from build123d import *

# Parameters (mm, degrees)
F0_W     = 150
F0_H     = 50
F1_DEPTH = 4
F3_D     = 5
F4_R     = 5
F5_SIZE  = 2


with BuildPart() as f1:
    # F0 (on Top) → F1 (new body)
    with BuildSketch(Plane.XY):
        Rectangle(F0_W, F0_H)
    extrude(amount=F1_DEPTH)

    # F3 (through all)
    with Locations(Plane.XY.offset(4)):
        with Locations((-56.25, 15), (-56.25, -15), (-18.75, -15), (-18.75, 15), (18.75, 15), (18.75, -15), (56.25, -15), (56.25, 15)):
            Hole(F3_D / 2)

    # F4
    f4_edges = [f1.edges().sort_by_distance(p)[0] for p in [
        (-75, 25, 2),
        (-75, -25, 2),
        (75, -25, 2),
        (75, 25, 2),
    ]]
    fillet(f4_edges, radius=F4_R)

    # F5
    f5_edges = [f1.edges().sort_by_distance(p)[0] for p in [
        (0, -25, 4),
    ]]
    chamfer(f5_edges, length=F5_SIZE)


solid = f1.part
Read the model definition and answer for the solid it produces. Units are mm, in the model's axes. Give positions to 0.01 mm unless a question says otherwise; leave off trailing zeros. Write each loop counter-clockwise with the first axis right and the second up, starting at its lowest first coordinate (ties: lowest second). Pieces come first, ordered by that corner, then holes. Notation, with made-up numbers: M 10,35.25 L 40,35.25 A23 cw 40,57.25 Z; hole C 80.25,16 d6. An arc over 180 degrees is marked long. One line per item, written item: value. Start each with the question number.
(1) Find the intervals of material crossed by line 1 (Y direction, x = -56, z = 1.8); line 2 (Y direction, x = 54.5, z = 3.4); line 3 (X direction, y = 3, z = 2.4), in increasing order.
(2) Determine the mould class of faces 1 (the conical face through (72.71, 22.65, 3.21)), 2 (the cylindrical face through (-74, -23, 1)), 3 (the cylindrical face through (-58.56, 14.04, 1.97)) for opening direction Y: pulls with the +Y half, pulls with the -Y half, needs draft (parallel to the pull), parting line crosses it, or undercut.
(3) Find section B-B (z = 2.75). Give the number of separate pieces and of enclosed holes in the cut face, plus the area to 3 significant figures.
(4) Find section A-A (x = -18.75). Determine the outline of the cut face in (y, z).
Results below:
1. line 1: y = -25 to -17.49, -12.51 to 12.51, 17.49 to 25
1. line 2: y = -23.6 to -16.79, -13.21 to 13.21, 16.79 to 23.6
1. line 3: x = -74.6 to 74.6
2. face 1: pulls with the +Y half
2. face 2: pulls with the -Y half
2. face 3: undercut
3. separate pieces: 1
3. enclosed holes: 8
3. area: 7,030 mm^2
4. outline: M -25,0 L -17.5,0 L -17.5,4 L -23,4 L -25,2 Z; M -12.5,0 L 12.5,0 L 12.5,4 L -12.5,4 Z; M 17.5,0 L 25,0 L 25,2 L 23,4 L 17.5,4 Z
